Build history of the part. All positions in model axes, mm. A direction names the side the tool comes from. Give positions to 0.01 mm unless a question says otherwise; leave off trailing zeros. Order: outer loops, then holes, each group sorted by start corner. A loop starts at its lowest first (then second) coordinate and runs counter-clockwise, first axis right, second up. Notation, with made-up numbers: M 75.25,2 L 111.25,2 A24 cw 111.25,37 Z; hole C -24,11 d1. An arc over 180 degrees is marked long. One line per item, written item: value.
from build123d import *

# Parameters (mm, degrees)
BOSS_EXTRUDE1_DEPTH   = 90
BOSS_EXTRUDE1_2_DEPTH = 90
SKETCH2_R             = 7.5
BOSS_EXTRUDE2_DEPTH   = 25
BOSS_EXTRUDE3_DEPTH   = 70
FILLET1_R             = 6
CUT_EXTRUDE1_DEPTH    = 18.5


with BuildPart() as part:
    # Sketch1 → Boss-Extrude1 (new body, symmetric)
    with BuildSketch(Plane(origin=(0, 0, 0), x_dir=(0, 0, -1), z_dir=(1, 0, 0))):
        Polygon((13, 17.5), (35, 17.5), (35, -1.5), (57.5, -1.5), (57.5, -17.5), (20, -17.5), (20, -2.5), (13, -2.5), align=None)
    extrude(amount=BOSS_EXTRUDE1_DEPTH, both=True)



with BuildPart() as body_2:
    # Sketch1 → Boss-Extrude1 2 (new body, symmetric)
    with BuildSketch(Plane(origin=(0, 0, 0), x_dir=(0, 0, -1), z_dir=(1, 0, 0))):
        Polygon((-13, -2.5), (-13, 17.5), (-35, 17.5), (-35, -1.5), (-57.5, -1.5), (-57.5, -17.5), (-20, -17.5), (-20, -2.5), align=None)
    extrude(amount=BOSS_EXTRUDE1_2_DEPTH, both=True)


with BuildPart() as part_1:
    add(part.part)

    add(body_2.part)  # Boss-Extrude2 merges body 2
    # Sketch2 → Boss-Extrude2 (add)
    with BuildSketch(Plane(origin=(90, 0, 0), x_dir=(0, 0, -1), z_dir=(1, 0, 0))):
        with BuildLine():
            Line((35, 17.5), (-35, 17.5))
            Line((-35, 17.5), (-35, 37.5))
            Line((-35, 37.5), (-15, 37.5))
            ThreePointArc((-15, 37.5), (0, 52.5), (15, 37.5))
            Line((15, 37.5), (35, 37.5))
            Line((35, 37.5), (35, 17.5))
        make_face()
        with Locations((0, 37.5)):
            Circle(SKETCH2_R, mode=Mode.SUBTRACT)
    extrude(amount=-BOSS_EXTRUDE2_DEPTH)

    # Sketch3 → Boss-Extrude3 (add)
    with BuildSketch(Plane(origin=(0, 0, -35), x_dir=(-1, 0, 0), z_dir=(0, 0, -1))):
        with BuildLine():
            Line((90, 17.5), (56, 17.5))
            Line((56, 17.5), (56, 62.5))
            Line((56, 62.5), (68, 62.5))
            ThreePointArc((68, 62.5), (84.115214431, 46.07043625), (90, 23.821840788))
            Line((90, 23.821840788), (90, 17.5))
        make_face()
    extrude(amount=-BOSS_EXTRUDE3_DEPTH)

    # Fillet1
    fillet1_edges = [part_1.edges().sort_by_distance(p)[0] for p in [
        (90, -9.5, -57.5),
        (-90, -9.5, 57.5),
        (90, -9.5, 57.5),
        (-90, -9.5, -57.5),
    ]]
    fillet(fillet1_edges, radius=FILLET1_R)

    # Sketch4 → Cut-Extrude1 (cut, through all)
    with BuildSketch(Plane(origin=(0, 0, 0), x_dir=(1, 0, 0), z_dir=(0, 1, 0))):
        with BuildLine():
            Line((7.5, 67.5), (7.5, 47.5))
            ThreePointArc((7.5, 47.5), (0, 40), (-7.5, 47.5))
            Line((-7.5, 47.5), (-7.5, 67.5))
            ThreePointArc((-7.5, 67.5), (0, 75), (7.5, 67.5))
        make_face()
        with BuildLine():
            Line((-7.5, -67.5), (-7.5, -47.5))
            ThreePointArc((-7.5, -47.5), (0, -40), (7.5, -47.5))
            Line((7.5, -47.5), (7.5, -67.5))
            ThreePointArc((7.5, -67.5), (0, -75), (-7.5, -67.5))
        make_face()
    extrude(amount=-CUT_EXTRUDE1_DEPTH, mode=Mode.SUBTRACT)


solid = part_1.part
1) Mould opens along Z. For faces 6 (the face through (-21, 17, 35)), 7 (the face through (7.5, -9, -53)), 8 (the face through (1, 7, 13)), 9 (the face through (0, -9, -40)) say: released by +Z, released by -Z, zero draft, split by the parting line, or undercut.
Check values:
face 6: released by +Z
face 7: zero draft
face 8: undercut
face 9: released by -Z
2) Saw through at A-A, the plane x = -51.5. Write the cut outline in (y, z).
Check values:
outline: M -17.5,-57.5 L -1.5,-57.5 L -1.5,-35 L 17.5,-35 L 17.5,-13 L -2.5,-13 L -2.5,-20 L -17.5,-20 Z; M -17.5,20 L -2.5,20 L -2.5,13 L 17.5,13 L 17.5,35 L -1.5,35 L -1.5,57.5 L -17.5,57.5 Z
3) Saw through at D-D, the plane x = 68. Write the cut outline in (y, z), then the cut area to 3 significant figures.
Check values:
outline: M -17.5,-57.5 L -1.5,-57.5 L -1.5,-35 L 37.5,-35 L 37.5,-15 A15 ccw 37.5,15 L 37.5,35 L -1.5,35 L -1.5,57.5 L -17.5,57.5 L -17.5,20 L -2.5,20 L -2.5,13 L 17.5,13 L 17.5,-13 L -2.5,-13 L -2.5,-20 L -17.5,-20 Z; hole C 37.5,0 d15
area: 3,630 mm^2
4) Saw through at B-B, the plane z = 0. Write the cut outline in (x, y), then the cut area to 3 significant figures.
Check values:
outline: M -90,17.5 L -56,17.5 L -56,62.5 L -68,62.5 A45 ccw -90,23.82 Z; M 65,17.5 L 90,17.5 L 90,30 L 65,30 Z; M 65,45 L 90,45 L 90,52.5 L 65,52.5 Z
area: 1,780 mm^2
5) Pin check, flat tips, straight feed: pin 1 (12 mm diameter, centred on x = -41.5, y = 18, fed in from +Z); pin 2 (2 mm diameter, centred on x = -25.5, z = 16.5, fed in from -Y); pin 3 (12 mm diameter, centred on x = -18, z = 2.5, fed in from -Y); pin 4 (11 mm diameter, centred on x = 31, z = 19, fed in from +Y). Stop position of each tip, or through.
Check values:
pin 1: z = 35
pin 2: y = -2.5
pin 3: through
pin 4: y = 17.5
6) Tool access for faces 1 (the face through (5, 17.5, 24)), 2 (the face through (-7.5, -9, -52)), 3 (the face through (78, 37.5, 25)), 4 (the face through (7.5, -9, 52)), 5 (the face through (1, 7, -13)): list every direction of +Z, -Z, +X, -X, +Y, -Y with a clear straight run to the whole face (end or side of a thin tool).
Check values:
face 1: +Z, -Z, +Y
face 2: -Z, +Y, -Y
face 3: +Z, +X, +Y
face 4: +Z, +Y, -Y
face 5: +X, -X, -Y
7) Drill centre lines: probe 1 along Y at (x, z) = (81.75, 0); probe 2 along Z at (x, y) = (81, 37); probe 3 along Y at (x, z) = (-10, -27). Where is each one in solid material? Low to high. Write a range as from..to.
Check values:
probe 1: 17.5..30, 45..52.5
probe 2: -35..-7.48, 7.48..35
probe 3: -17.5..17.5
8) Saw through at C-C, the plane y = 20. Write the cut outline in (x, z), then the cut area to 3 significant figures.
Check values:
outline: M -90,-35 L -56,-35 L -56,35 L -90,35 Z; M 65,-35 L 90,-35 L 90,35 L 65,35 Z
area: 4,130 mm^2
